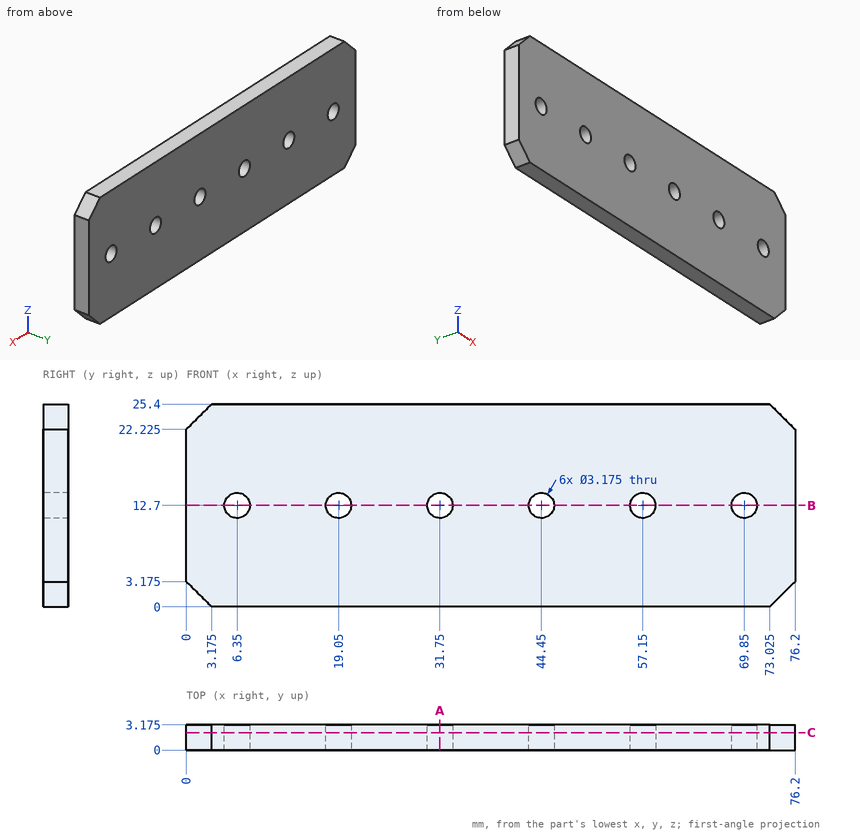
Here's the drawing with two shaded views (mm, measured from the low corner). I have some questions. Give positions to 0.01 mm unless a question says otherwise; leave off trailing zeros. Order: outer loops, then holes, each group sorted by start corner. A loop starts at its lowest first (then second) coordinate and runs counter-clockwise, first axis right, second up. Notation, with made-up numbers: (-7.75, 54.25) - (51.25, 54.25) arc R10 cw to (51.25, 65.25) - close; hole circle Ø10 at (62, -27.75). An arc over 180 degrees is marked (long way). Write each question's results on one line, items separated by ' | '.
1) Suppose I cut it at A-A, the plane x = 31.75. Write out the boundary of the cut face in (y, z) (1 decimal).
Final values:
outline: (0, 0) - (3.2, 0) - (3.2, 11.1) - (0, 11.1) - close; (0, 14.3) - (3.2, 14.3) - (3.2, 25.4) - (0, 25.4) - close
2) Suppose I cut it at B-B, the plane z = 12.7. Write out the boundary of the cut face in (x, y) (1 decimal), then the cut area to 3 significant figures.
Final values:
outline: (0, 0) - (4.8, 0) - (4.8, 3.2) - (0, 3.2) - close; (7.9, 0) - (17.5, 0) - (17.5, 3.2) - (7.9, 3.2) - close; (20.6, 0) - (30.2, 0) - (30.2, 3.2) - (20.6, 3.2) - close; (33.3, 0) - (42.9, 0) - (42.9, 3.2) - (33.3, 3.2) - close; (46, 0) - (55.6, 0) - (55.6, 3.2) - (46, 3.2) - close; (58.7, 0) - (68.3, 0) - (68.3, 3.2) - (58.7, 3.2) - close; (71.4, 0) - (76.2, 0) - (76.2, 3.2) - (71.4, 3.2) - close | area: 181 mm^2
3) Suppose I cut it at C-C, the plane y = 2.2. Give the number of separate pieces and of enclosed holes in the cut face, then the cut area to 3 significant figures.
Final values:
separate pieces: 1 | enclosed holes: 6 | area: 1,870 mm^2
4) Please list where these lines run through material, in increasing order: line 1 along Z through (x, y) = (44.45, 1.8); line 2 along Z through (x, y) = (43, 1.6); line 3 along X through (y, z) = (0.45, 2.25) (3 decimals). Write a range as [from, to].
Final values:
line 1: z = [0, 11.11], [14.29, 25.4] | line 2: z = [0, 12.05], [13.35, 25.4] | line 3: x = [0.925, 75.275]
